Here's how the part is built. I have some questions about the finished solid (model axes, mm). Round coordinates to 2 decimals unless told otherwise and drop trailing zeros. Write each loop counter-clockwise with the first axis right and the second up, starting at its lowest first coordinate (ties: lowest second). Pieces come first, ordered by that corner, then holes. Notation, with made-up numbers: (26.5, -7.5) -> (47.5, -7.5) arc R15 ccw to (47.5, 3.5) -> close; hole circle Ø5 at (-20, 31.5). An arc over 180 degrees is marked (long way). Put each result on its own line as item: value. Start each with the question number.
1. We'd pull the mould along X, two halves only. Please class faces 1 (the face through (0, 6, -25.4)), 2 (the face through (0.628, 7.691, -14.274)), 3 (the face through (25.4, 6, 0)): +X half, -X half, draft (parallel to the pull), parting line (faces both ways), or undercut.
2. Suppose I cut it at C-C (y = 10.25). Please give me the cut outline in (x, z) (1 decimal), then the cut area to 3 significant figures.
3. For pin 1 (2 mm diameter, centred on x = 11, z = -13.5, fed in from -Y), with a flat end and sliding along its axis, tell me the tip position at first contact or that it passes through.
4. Suppose I cut it at B-B (x = 0). Please give me the cut outline in (y, z), then the cut area to 3 significant figures.
5. I need wall thicknesses on probe 1 along X at (y, z) = (10.75, 0); probe 2 along X at (y, z) = (1, 8); probe 3 along Z at (x, y) = (12.5, 6.5). Which ranges of each line are inside material? Lowest first, please. Write a range as from..to.
6. Suppose I cut it at A-A (z = 0). Please give me the cut outline in (x, y), then the cut area to 3 significant figures.
```python
from build123d import *

# Parameters (mm, degrees)
SKETCH1_W           = 50.8
SKETCH1_H           = 50.8
BOSS_EXTRUDE1_DEPTH = 12.7
CUT_EXTRUDE1_REACH  = 40.1
SKETCH2_R           = 14.2875
CHAMFER1_SIZE       = 2.54


with BuildPart() as part:
    # Sketch1 → Boss-Extrude1 (new body)
    with BuildSketch(Plane(origin=(0, 0, 0), x_dir=(1, 0, 0), z_dir=(0, 1, 0))):
        Rectangle(SKETCH1_W, SKETCH1_H)
    extrude(amount=BOSS_EXTRUDE1_DEPTH)

    # Sketch2 → Cut-Extrude1 (cut, up to next)
    with BuildSketch(Plane(origin=(0, 12.7, 0), x_dir=(1, 0, 0), z_dir=(0, 1, 0)), mode=Mode.PRIVATE) as cut_extrude1_sk1:
        with Locations(Location((0, 0, 0), (0, 0, 270))):
            Circle(SKETCH2_R)
    cut_extrude1_tool1 = extrude(cut_extrude1_sk1.sketch, amount=-CUT_EXTRUDE1_REACH, mode=Mode.PRIVATE) & part.part
    add(cut_extrude1_tool1.solids().sort_by_distance((0, 12.7, 0))[0], mode=Mode.SUBTRACT)

    # Chamfer1
    chamfer1_edges = [part.edges().sort_by_distance(p)[0] for p in [
        (0, 0, -14.2875),
    ]]
    chamfer(chamfer1_edges, length=CHAMFER1_SIZE)


solid = part.part
```
Verdict:
1. face 1: draft
1. face 2: undercut
1. face 3: +X half
2. outline: (-25.4, -25.4) -> (25.4, -25.4) -> (25.4, 25.4) -> (-25.4, 25.4) -> close; hole circle Ø28.6 at (0, 0)
2. area: 1,940 mm^2
3. pin 1: stops at y = 0
4. outline: (0, -25.4) -> (12.7, -25.4) -> (12.7, -14.29) -> (2.54, -14.29) -> (0, -16.83) -> close; (0, 16.83) -> (2.54, 14.29) -> (12.7, 14.29) -> (12.7, 25.4) -> (0, 25.4) -> close
4. area: 276 mm^2
5. probe 1: x = -25.4..-14.29, 14.29..25.4
5. probe 2: x = -25.4..-13.66, 13.66..25.4
5. probe 3: z = -25.4..-6.92, 6.92..25.4
6. outline: (-25.4, 0) -> (-16.83, 0) -> (-14.29, 2.54) -> (-14.29, 12.7) -> (-25.4, 12.7) -> close; (14.29, 2.54) -> (16.83, 0) -> (25.4, 0) -> (25.4, 12.7) -> (14.29, 12.7) -> close
6. area: 276 mm^2
